Geometry check sheet. Reference: the model listing, model coordinates, mm. A direction names the side the tool comes from. Coordinates: 2 decimals unless noted, no trailing zeros. Write each loop counter-clockwise with the first axis right and the second up, starting at its lowest first coordinate (ties: lowest second). Pieces come first, ordered by that corner, then holes. Notation, with made-up numbers: M -10.5,76 L 43.5,76 A24 cw 43.5,102 Z; hole C -34,46 d10. An arc over 180 degrees is marked long. Answer as a JSON object with one key per item and string values. Group by question number.
```python
from build123d import *

# Parameters (mm, degrees)
SALIENTE_EXTRUIR1_DEPTH = 6
CORTAR_EXTRUIR2_DEPTH   = 10
SALIENTE_EXTRUIR2_REACH = 33.971
CROQUIS3_R              = 1.5
SALIENTE_EXTRUIR3_START = 10
SALIENTE_EXTRUIR3_DEPTH = 6
CROQUIS5_R              = 1.9
CORTAR_EXTRUIR3_DEPTH   = 6
CORTAR_EXTRUIR4_DEPTH   = 10
CORTAR_EXTRUIR8_DEPTH   = 10


with BuildPart() as part:
    # Croquis1 → Saliente-Extruir1 (new body)
    with BuildSketch(Plane.XY):
        with BuildLine():
            Line((-26.569033706, 2.264395111), (-54.029300138, 14.344700052))
            ThreePointArc((-54.029300138, 14.344700052), (-27.848836662, 23.896462082), (0, 24.942942963))
            Line((0, 24.942942963), (0, -0.057057037))
            add(Edge.make_bspline(
                [(-26.569033706, 2.264395111), (-17.747364857, 14.365738672), (0, -0.057057037)],
                knots=[0, 0, 0, 1, 1, 1], degree=2))
        make_face()
    extrude(amount=SALIENTE_EXTRUIR1_DEPTH)

    # Croquis2 → Cortar-Extruir2 (cut)
    with BuildSketch(Plane.XY.offset(6)):
        Polygon((-43.045193565, 9.512578075), (-39.823778914, 16.835315791), (-28.839672341, 12.003193814), (-32.061086993, 4.680456099), align=None)
    extrude(amount=-CORTAR_EXTRUIR2_DEPTH, mode=Mode.SUBTRACT)

    # Croquis3 → Saliente-Extruir2 (add, up to next)
    with BuildSketch(Plane(origin=(-28.587581395, 12.576232705, 0), x_dir=(0, 0, 1), z_dir=(-0.915342214401337, 0.4026768313857366, 0)), mode=Mode.PRIVATE) as saliente_extruir2_sk1:
        with Locations(Location((3, -4.626037871, 0), (0, 0, 90))):
            Circle(CROQUIS3_R)
    saliente_extruir2_tool1 = extrude(saliente_extruir2_sk1.sketch, amount=SALIENTE_EXTRUIR2_REACH, mode=Mode.PRIVATE) - part.part
    add(saliente_extruir2_tool1.solids().sort_by_distance((-30.45038, 8.341825, 3))[0])

    # Croquis4 → Saliente-Extruir3 (add)
    with BuildSketch(Plane(origin=(0, 0, 0), x_dir=(1, 0, 0), z_dir=(0, 1, 0)).offset(SALIENTE_EXTRUIR3_START)):
        with BuildLine():
            Line((0, 0), (4, 0))
            ThreePointArc((4, 0), (7, -3), (4, -6))
            Line((4, -6), (0, -6))
            Line((0, -6), (0, 0))
        make_face()
    extrude(amount=SALIENTE_EXTRUIR3_DEPTH)

    # Croquis5 → Cortar-Extruir3 (cut)
    with BuildSketch(Plane(origin=(0, 16, 0), x_dir=(1, 0, 0), z_dir=(0, 1, 0))):
        with Locations(Location((4, -3, 0), (0, 0, 270))):
            Circle(CROQUIS5_R)
    extrude(amount=-CORTAR_EXTRUIR3_DEPTH, mode=Mode.SUBTRACT)

    # Croquis6 → Cortar-Extruir4 (cut)
    with BuildSketch(Plane.XY.offset(6)):
        Polygon((-54.217314507, 14.240228789), (-26.345009663, 1.686933832), (-25.374680505, 3.841372979), (-53.24698535, 16.394667936), align=None)
    extrude(amount=-CORTAR_EXTRUIR4_DEPTH, mode=Mode.SUBTRACT)

    # Croquis7 → Cortar-Extruir8 (cut)
    with BuildSketch(Plane.XY.offset(6)):
        with BuildLine():
            Line((-44.469656668, 18.924767513), (-48.553751341, 14.280901201))
            ThreePointArc((-48.553751341, 14.280901201), (-47.473480209, 17.448678059), (-44.469656668, 18.924767513))
        make_face()
    extrude(amount=-CORTAR_EXTRUIR8_DEPTH, mode=Mode.SUBTRACT)


with BuildPart() as body_2:
    # of the pieces the cut leaves, the one that is kept (cortar_extruir8_keep)
    add(part.part.solids().sort_by_distance((0, 24.942942963, 0))[0])


solid = body_2.part
```
1) Section check A-A (y = 12.75). State how many separate pieces and enclosed holes the cut face has, then the cut area to 3 significant figures.
2) Set-up check for faces 1 (the flat face through (0, 21, 3)), 2 (the flat face through (0, 5, 3)), 3 (the flat face through (-34.409, 14.453, 3.042)), 4 (the flat face through (-29.765, 9.899, 3.042)), 5 (the cylindrical face through (7, 13, 3)): record each of +Z, -Z, +X, -X, +Y, -Y from which the full face is reachable in a straight line by a thin tool's end or side.
3) Go/stop test with flat-tipped pins: pin 1 Ø1.5 at (y, z) = (22, 4.5) entering from +X; pin 2 Ø3 at (x, z) = (4, 2.5) entering from +Y; pin 3 Ø3 at (x, z) = (2, 2) entering from -Y; pin 4 Ø8 at (x, y) = (-13, 16.5) entering from -Z. Record where each tip stops, or that it passes through.
4) Section check C-C (y = 23.5). Record the cut outline in (x, z).
5) Draft check along X on faces 6 (the flat face through (2, 16, 2)), 7 (the cylindrical face through (-22.93, 24.72, 2.96)), 8 (the flat face through (-40.767, 14.692, 3.042)). Enter one of: +X half, -X half, draft (parallel to the pull), parting line (faces both ways), or undercut.
6) Material ranges on probe 1 along X at (y, z) = (11, 3.75); probe 2 along X at (y, z) = (14.5, 2); probe 3 along X at (y, z) = (5, 4.25), recorded low to high. Write a range as [from, to].
Entries:
{
 "1": {"separate pieces": "2", "enclosed holes": "1", "area": "243 mm^2"},
 "2": {"face 1": "+Z, -Z, +X, +Y", "face 2": "+Z, -Z, +X, -Y", "face 3": "+Z, -Z", "face 4": "none", "face 5": "+X, +Y, -Y"},
 "3": {"pin 1": "x = 0", "pin 2": "y = 16", "pin 3": "y = 10", "pin 4": "z = 0"},
 "4": {"outline": "M -29.76,0 L 0,0 L 0,6 L -29.76,6 Z"},
 "5": {"face 6": "draft", "face 7": "parting line", "face 8": "undercut"},
 "6": {"probe 1": "[-39.72, -33.27], [-29.28, 2.25], [5.75, 6.9]", "probe 2": "[-48.36, -40.85], [-34.52, 2.38], [5.62, 6.83]", "probe 3": "[-27.95, -24.08], [-7.37, 0]"}
}
